Here's how the part is built. I have some questions about the finished solid (model axes, mm). Coordinates: 2 decimals unless noted, no trailing zeros.
Item 1: If I drill on line 1 (Y direction, x = 139, z = 14); line 2 (Y direction, x = 292.1, z = 12.5), over which ranges is the centre line in solid material (lowest first)?
Item 2: I'm going to push a flat-ended pin straight in: pin 1 Ø2.5 at (x, y) = (24.5, -22) entering from +Z. Where does the tip first touch, or does it pass through?
Item 3: If we section it at A-A (z = 10.25): Count the separate pieces of the cut face and the enclosed holes in it, then the cut area to 3 significant figures.
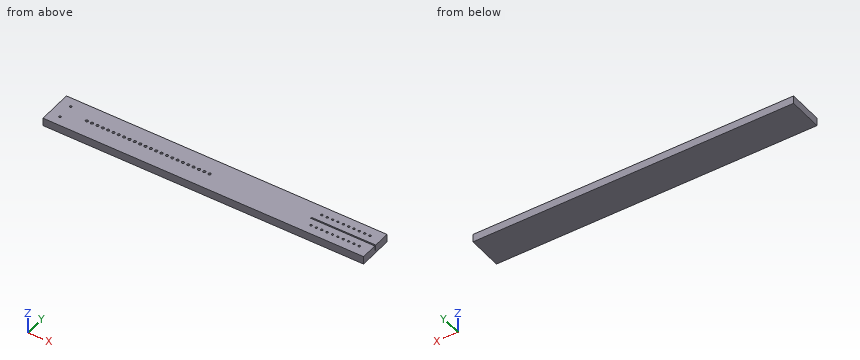
from build123d import *

# Parameters (mm, degrees)
F0_W     = 762
F0_H     = 82.55
F1_DEPTH = 19.05
F2_R     = 2.5
F2_R_2   = 3.175
F2_W     = 152.4
F2_H     = 3.175
F3_DEPTH = 12.7


with BuildPart() as f1:
    # F0 (on Top) → F1 (new body)
    with BuildSketch(Plane.XY):
        with Locations((381, -41.275)):
            Rectangle(F0_W, F0_H)
    extrude(amount=F1_DEPTH)

    # F2 (on face) → F3 (cut)
    with BuildSketch(Plane.XY.offset(19.05)):
        with Locations((25.4, -22.225)):
            Circle(F2_R)
        with Locations((25.4, -60.325)):
            Circle(F2_R)
        with Locations((76.2, -41.275)):
            Circle(F2_R_2)
        with Locations((736.6, -22.225)):
            Circle(F2_R)
        with Locations((736.6, -60.325)):
            Circle(F2_R)
        with Locations((88.9, -41.275)):
            Circle(F2_R_2)
        with Locations((101.6, -41.275)):
            Circle(F2_R_2)
        with Locations((114.3, -41.275)):
            Circle(F2_R_2)
        with Locations((127, -41.275)):
            Circle(F2_R_2)
        with Locations((139.7, -41.275)):
            Circle(F2_R_2)
        with Locations((152.4, -41.275)):
            Circle(F2_R_2)
        with Locations((165.1, -41.275)):
            Circle(F2_R_2)
        with Locations((177.8, -41.275)):
            Circle(F2_R_2)
        with Locations((190.5, -41.275)):
            Circle(F2_R_2)
        with Locations((203.2, -41.275)):
            Circle(F2_R_2)
        with Locations((215.9, -41.275)):
            Circle(F2_R_2)
        with Locations((723.9, -22.225)):
            Circle(F2_R)
        with Locations((723.9, -60.325)):
            Circle(F2_R)
        with Locations((711.2, -22.225)):
            Circle(F2_R)
        with Locations((711.2, -60.325)):
            Circle(F2_R)
        with Locations((698.5, -22.225)):
            Circle(F2_R)
        with Locations((698.5, -60.325)):
            Circle(F2_R)
        with Locations((685.8, -22.225)):
            Circle(F2_R)
        with Locations((685.8, -60.325)):
            Circle(F2_R)
        with Locations((673.1, -22.225)):
            Circle(F2_R)
        with Locations((673.1, -60.325)):
            Circle(F2_R)
        with Locations((660.4, -22.225)):
            Circle(F2_R)
        with Locations((660.4, -60.325)):
            Circle(F2_R)
        with Locations((647.7, -22.225)):
            Circle(F2_R)
        with Locations((647.7, -60.325)):
            Circle(F2_R)
        with Locations((635, -22.225)):
            Circle(F2_R)
        with Locations((635, -60.325)):
            Circle(F2_R)
        with Locations((685.8, -41.275)):
            Rectangle(F2_W, F2_H)
        with Locations((622.3, -22.225)):
            Circle(F2_R)
        with Locations((622.3, -60.325)):
            Circle(F2_R)
        with Locations((228.6, -41.275)):
            Circle(F2_R_2)
        with Locations((241.3, -41.275)):
            Circle(F2_R_2)
        with Locations((254, -41.275)):
            Circle(F2_R_2)
        with Locations((266.7, -41.275)):
            Circle(F2_R_2)
        with Locations((279.4, -41.275)):
            Circle(F2_R_2)
        with Locations((292.1, -41.275)):
            Circle(F2_R_2)
        with Locations((304.8, -41.275)):
            Circle(F2_R_2)
        with Locations((317.5, -41.275)):
            Circle(F2_R_2)
        with Locations((330.2, -41.275)):
            Circle(F2_R_2)
        with Locations((342.9, -41.275)):
            Circle(F2_R_2)
        with Locations((355.6, -41.275)):
            Circle(F2_R_2)
        with Locations((368.3, -41.275)):
            Circle(F2_R_2)
    extrude(amount=-F3_DEPTH, mode=Mode.SUBTRACT)


solid = f1.part
Answer list:
1. line 1: y = -82.55 to -44.37, -38.18 to 0
1. line 2: y = -82.55 to -44.45, -38.1 to 0
2. pin 1: stops at z = 6.35
3. separate pieces: 1
3. enclosed holes: 46
3. area: 61,200 mm2
